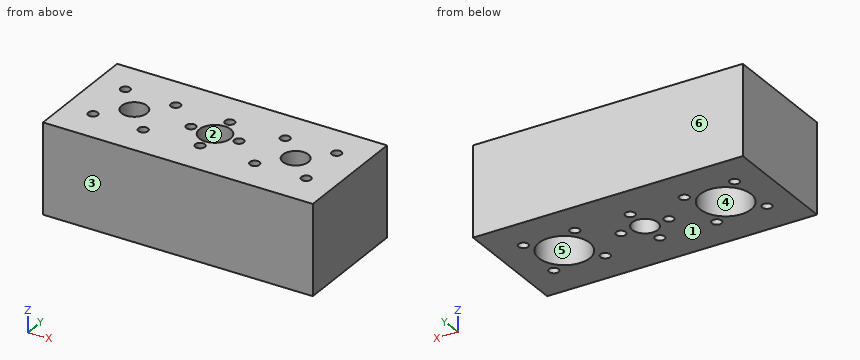
from build123d import *

# Parameters (mm, degrees)
SKETCH_1_W            = 90
SKETCH_1_H            = 40
EXTRUDE_1_DEPTH       = 30
HOLE_WIZARD_356_D     = 8.5
HOLE_WIZARD_461_D     = 10.4
HOLE_WIZARD_461_DEPTH = 12
HOLE_WIZARD_561_D     = 3.2
HOLE_WIZARD_727_D     = 8.5
HOLE_WIZARD_831_D     = 3.2
HOLE_WIZARD_989_D     = 17
HOLE_WIZARD_989_DEPTH = 20


with BuildPart() as part:
    # 草图1 → 凸台-拉伸1 (new body)
    with BuildSketch(Plane.XY):
        Rectangle(SKETCH_1_W, SKETCH_1_H)
    extrude(amount=EXTRUDE_1_DEPTH)

    # Hole Wizard 356 (through all)
    with Locations(Plane.XY.offset(30)):
        with Locations((0, 0)):
            Hole(HOLE_WIZARD_356_D / 2)

    # Hole Wizard 461
    with Locations(Plane.XY.offset(30)):
        with Locations((0, 0)):
            Hole(HOLE_WIZARD_461_D / 2, depth=HOLE_WIZARD_461_DEPTH)

    # Hole Wizard 561 (through all)
    with Locations(Plane.XY.offset(30)):
        with Locations((8, 0), (0, 8), (-8, 0), (0, -8)):
            Hole(HOLE_WIZARD_561_D / 2)

    # Hole Wizard 727 (through all)
    with Locations(Plane(origin=(0, 0, 0), x_dir=(-1, 0, 0), z_dir=(0, 0, -1))):
        with Locations((-26.909213315, 0)):
            hole_wizard_727 = Hole(HOLE_WIZARD_727_D / 2)

    # Hole Wizard 831 (through all)
    with Locations(Plane(origin=(0, 0, 0), x_dir=(-1, 0, 0), z_dir=(0, 0, -1))):
        with Locations((-18.261181521, 8.319347696), (-35.228561011, 8.648031794), (-35.557245109, -8.319347696), (-18.589865619, -8.648031794)):
            hole_wizard_831 = Hole(HOLE_WIZARD_831_D / 2)

    # Hole Wizard 989
    with Locations(Plane(origin=(0, 0, 0), x_dir=(-1, 0, 0), z_dir=(0, 0, -1))):
        with Locations((-26.909213315, 0)):
            hole_wizard_989 = Hole(HOLE_WIZARD_989_D / 2, depth=HOLE_WIZARD_989_DEPTH)

    # 镜向1: Hole Wizard 727, Hole Wizard 831, Hole Wizard 989 across plane
    add(hole_wizard_727.mirror(Plane.ZY), mode=Mode.SUBTRACT)
    add(hole_wizard_831.mirror(Plane.ZY), mode=Mode.SUBTRACT)
    add(hole_wizard_989.mirror(Plane.ZY), mode=Mode.SUBTRACT)


solid = part.part
Part model, mm, in its own coordinate system. Face numbers are marked on the shaded views. A direction names the side the tool comes from. Round coordinates to 2 decimals unless told otherwise and drop trailing zeros. Loops run counter-clockwise (first coordinate to the right, second up) from the corner with the lowest first, then second, coordinate; pieces in that order, holes last. Notation, with made-up numbers: (-39.5, 2) - (-23.5, 2) arc R22 ccw to (-23.5, 29) - close; hole circle Ø7 at (83, 86). An arc over 180 degrees is marked (long way). Answer as a JSON object with one key per item and string values.
Item 1: Band-saw the part on B-B on y = 3. List the corners of the cut face in (x, z), plus the area to 3 significant figures.
Output:
{"outline": "(-45, 0) - (-34.86, 0) - (-34.86, 20) - (-29.92, 20) - (-29.92, 30) - (-45, 30) - close; (-23.9, 20) - (-18.96, 20) - (-18.96, 0) - (-3.01, 0) - (-3.01, 18) - (-4.25, 18) - (-4.25, 30) - (-23.9, 30) - close; (3.01, 0) - (18.96, 0) - (18.96, 20) - (23.9, 20) - (23.9, 30) - (4.25, 30) - (4.25, 18) - (3.01, 18) - close; (29.92, 20) - (34.86, 20) - (34.86, 0) - (45, 0) - (45, 30) - (29.92, 30) - close", "area": "1,730 mm2"}
Item 2: Tool access for the marked faces 5 and 6: list every direction of +Z, -Z, +X, -X, +Y, -Y with a clear straight run to the whole face (end or side of a thin tool).
Output:
{"face 5": "-Z", "face 6": "+Z, -Z, +X, -X, +Y"}
Item 3: Wall check: L1, parallel to X at y = 1, z = 12.25; L2, parallel to X at y = -10, z = 20.25; L3, parallel to Y at x = 0, z = 7.25. Give the ranges that are in metal, low to high.
Output:
{"L1": "-45 to -35.35, -18.47 to -9.25, -6.75 to -4.13, 4.13 to 6.75, 9.25 to 18.47, 35.35 to 45", "L2": "-45 to -19.45, -17.73 to 17.73, 19.45 to 45", "L3": "-20 to -9.6, -6.4 to -4.25, 4.25 to 6.4, 9.6 to 20"}
Item 4: Band-saw the part on A-A on x = 0. List the corners of the cut face in (y, z).
Output:
{"outline": "(-20, 0) - (-9.6, 0) - (-9.6, 30) - (-20, 30) - close; (-6.4, 0) - (-4.25, 0) - (-4.25, 18) - (-5.2, 18) - (-5.2, 30) - (-6.4, 30) - close; (4.25, 0) - (6.4, 0) - (6.4, 30) - (5.2, 30) - (5.2, 18) - (4.25, 18) - close; (9.6, 0) - (20, 0) - (20, 30) - (9.6, 30) - close"}
Item 5: Pull direction Y, two halves, no side cores. Call the marked faces 1, 2, 3 and 4: pulls with the +Y half, pulls with the -Y half, needs draft (parallel to the pull), parting line crosses it, or undercut.
Output:
{"face 1": "needs draft", "face 2": "undercut", "face 3": "pulls with the -Y half", "face 4": "undercut"}
Item 6: Pin check, flat tips, straight feed: pin 1 (7.5 mm diameter, centred on x = -26.91, y = 0, fed in from -Z); pin 2 (5 mm diameter, centred on x = 31, y = 0.5, fed in from -Z). Stop position of each tip, or through.
Output:
{"pin 1": "through", "pin 2": "z = 20"}
Item 7: Band-saw the part on C-C on z = 6. State how many separate pieces and enclosed holes the cut face has, plus the area to 3 significant figures.
Output:
{"separate pieces": "1", "enclosed holes": "15", "area": "2,990 mm2"}
